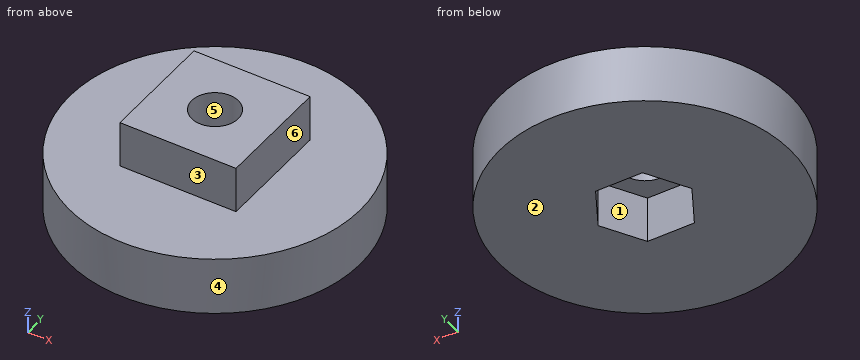
Autodesk Inventor part; units mm, degrees
ref_plane "YZ Plane" through (0, 0, 0) normal (1, 0, 0) x (0, 1, 0)
ref_plane "XZ Plane" through (0, 0, 0) normal (0, 1, 0) x (-1, 0, 0)
ref_plane "XY Plane" through (0, 0, 0) normal (0, 0, 1) x (1, 0, 0)
sketch "Sketch1" plane through (0, 0, 0) normal (0, 0, 1) x (1, 0, 0)
  circle A0 centre (0, 0) radius 12.5
  dimension "d0" = 25
extrude "Extrusion1" add sketch "Sketch1" along normal blind 5
sketch "Sketch2" plane through (0, 0, 5) normal (0, 0, 1) x (1, 0, 0)
  circle A0 centre (0, 0) radius 12.5
  circle A1 centre (0, 0) radius 2
  dimension "d4" = 4
extrude "Extrusion2" cut sketch "Sketch2" against normal blind 5 contours A1
sketch "Sketch3" plane through (0, 0, 5) normal (0, 0, 1) x (1, 0, 0)
  circle A0 centre (0, 0) radius 2
  line L0 (-5, -5) -> (5, -5)
  line L1 (5, -5) -> (5, 5)
  line L2 (5, 5) -> (-5, 5)
  line L3 (-5, 5) -> (-5, -5)
  dimension "d8" = 10
  dimension "d10" = 10
  dimension "d11" = 5
  dimension "d12" = 5
extrude "Extrusion3" add sketch "Sketch3" along normal blind 4
sketch "Sketch4" plane through (0, 0, 0) normal (0, 0, -1) x (-1, 0, 0)
  circle A0 centre (0, 0) radius 2
  circle A1 centre (0, 0) radius 12.5
  line L0 (-2.023, 3.4987) -> (2.0185, 3.5013)
  line L1 (2.0185, 3.5013) -> (4.0415, 0.0026)
  line L2 (4.0415, 0.0026) -> (2.023, -3.4987)
  line L3 (2.023, -3.4987) -> (-2.0185, -3.5013)
  line L4 (-2.0185, -3.5013) -> (-4.0415, -0.0026)
  line L5 (-4.0415, -0.0026) -> (-2.023, 3.4987)
  dimension "d15" = 7
extrude "Extrusion4" cut sketch "Sketch4" against normal blind 4 contours L0 L1 L2 L3 L4 L5
properties part number "Tension Push washer backplate"
The model under review builds one solid part; all positions refer to its coordinate system, in mm. Face numbers are marked on the shaded views. A direction names the side the tool comes from. Coordinates: 2 decimals unless noted, no trailing zeros. Write each loop counter-clockwise with the first axis right and the second up, starting at its lowest first coordinate (ties: lowest second). Pieces come first, ordered by that corner, then holes. Notation, with made-up numbers: M -36.75,41 L 7.25,41 A35 ccw 7.25,75 Z; hole C 6,60.5 d3. An arc over 180 degrees is marked long. Put each result on its own line as item: value.
1) Add section C-C on y = -1.25. Give the boundary of the cut face in (x, z), then the cut area to 3 significant figures.
Computed:
outline: M -12.44,0 L -3.32,0 L -3.32,4 L -1.56,4 L -1.56,9 L -5,9 L -5,5 L -12.44,5 Z; M 1.56,4 L 3.32,4 L 3.32,0 L 12.44,0 L 12.44,5 L 5,5 L 5,9 L 1.56,9 Z
area: 122 mm2
2) Clearance check with flat-ended pins moving along their axes: pin 1 Ø2 at (y, z) = (0.5, 7.5) entering from -X; pin 2 Ø3 at (x, z) = (-1, 7) entering from +Y; pin 3 Ø5 at (x, z) = (7.5, 5.5) entering from +Y. State where each tip first meets the part, or that it passes through.
Computed:
pin 1: stops at x = -5
pin 2: stops at y = 5
pin 3: stops at y = 11.43
3) Add section D-D on z = 1. Give the boundary of the cut face in (x, y).
Computed:
outline: C 0,0 d25; hole M -4.04,0 L -2.02,-3.5 L 2.02,-3.5 L 4.04,0 L 2.02,3.5 L -2.02,3.5 Z
4) Wall thickness on probe 1 along X at (y, z) = (0, 5.15); probe 2 along Z at (x, y) = (-10, 7): over which ranges is each line inside the solid? List them lowest first. Write a range as [from, to].
Computed:
probe 1: x = [-5, -2], [2, 5]
probe 2: z = [0, 5]
5) Add section B-B on z = 8.5. Give the boundary of the cut face in (x, y), then the cut area to 3 significant figures.
Computed:
outline: M -5,-5 L 5,-5 L 5,5 L -5,5 Z; hole C 0,0 d4
area: 87.4 mm2
6) Draft analysis for pull direction Y (two halves, no side actions). For the marked faces 4, 5 and 6, state which applies: released by +Y, released by -Y, zero draft, split by the parting line, or undercut.
Computed:
face 4: split by the parting line
face 5: undercut
face 6: zero draft
7) Add section A-A on x = 0. Give the boundary of the cut face in (y, z), then the cut area to 3 significant figures.
Computed:
outline: M -12.5,0 L -3.5,0 L -3.5,4 L -2,4 L -2,9 L -5,9 L -5,5 L -12.5,5 Z; M 2,4 L 3.5,4 L 3.5,0 L 12.5,0 L 12.5,5 L 5,5 L 5,9 L 2,9 Z
area: 117 mm2
8) For the marked faces 1, 2 and 3, list the 3-axis set-ups (+Z, -Z, +X, -X, +Y, -Y) from which the entire face can be reached by the end or side of a thin tool; tool diameter is ignored.
Computed:
face 1: -Z
face 2: -Z, +X, -X, +Y, -Y
face 3: +Z, +X, -X, -Y
